Design review of the part built by this model. Coordinates are the model's own, in mm. A direction names the side the tool comes from. Coordinates: 2 decimals unless noted, no trailing zeros. Write each loop counter-clockwise with the first axis right and the second up, starting at its lowest first coordinate (ties: lowest second). Pieces come first, ordered by that corner, then holes. Notation, with made-up numbers: (-14.75, -30) - (-9.75, -30) arc R26 cw to (-9.75, 6) - close; hole circle Ø5 at (58, 17). An arc over 180 degrees is marked (long way). One line per item, written item: value.
from build123d import *

# Parameters (mm, degrees)
F0_R     = 10.16
F1_DEPTH = 15.7734
F3_DEPTH = 25.4
F4_R     = 5.08


with BuildPart() as f1:
    # F0 (on Top) → F1 (new body)
    with BuildSketch(Plane.XY):
        with BuildLine():
            ThreePointArc((5.0426470588, -28.1265414802), (21.9160245563, -18.3362616868), (28.575, 0))
            ThreePointArc((28.575, 0), (21.9160245563, 18.3362616868), (5.0426470588, 28.1265414802))
            ThreePointArc((5.0426470588, 28.1265414802), (-28.575, 0), (5.0426470588, -28.1265414802))
        make_face()
        with BuildLine():
            ThreePointArc((13.4477648793, -4.826), (-14.2875, 0), (13.4477648793, 4.826))
            Line((13.4477648793, 4.826), (18.5293, 4.826))
            Line((18.5293, 4.826), (18.5293, -4.826))
            Line((18.5293, -4.826), (13.4477648793, -4.826))
        make_face(mode=Mode.SUBTRACT)
        with BuildLine():
            ThreePointArc((5.0426470588, 28.1265414802), (21.9160245563, 18.3362616868), (28.575, 0))
            ThreePointArc((28.575, 0), (21.9160245563, -18.3362616868), (5.0426470588, -28.1265414802))
            Line((5.0426470588, -28.1265414802), (57.3367647059, -18.7510276535))
            ThreePointArc((57.3367647059, -18.7510276535), (73.025, 0), (57.3367647059, 18.7510276535))
            Line((57.3367647059, 18.7510276535), (5.0426470588, 28.1265414802))
        make_face()
        with Locations((53.975, 0)):
            Circle(F0_R, mode=Mode.SUBTRACT)
    extrude(amount=F1_DEPTH)

    # F2 (on face) → F3 (join)
    with BuildSketch(Plane.XY.offset(15.7734)):
        with BuildLine():
            ThreePointArc((5.0426470588, -28.1265414802), (21.9160245563, -18.3362616868), (28.575, 0))
            ThreePointArc((28.575, 0), (21.9160245563, 18.3362616868), (5.0426470588, 28.1265414802))
            ThreePointArc((5.0426470588, 28.1265414802), (-28.575, 0), (5.0426470588, -28.1265414802))
        make_face()
        with BuildLine():
            Line((18.5293, -4.826), (13.4477648793, -4.826))
            ThreePointArc((13.4477648793, -4.826), (-14.2875, 0), (13.4477648793, 4.826))
            Line((13.4477648793, 4.826), (18.5293, 4.826))
            Line((18.5293, 4.826), (18.5293, -4.826))
        make_face(mode=Mode.SUBTRACT)
    extrude(amount=F3_DEPTH)

    # F4
    f4_edges = [f1.edges().sort_by_distance(p)[0] for p in [
        (-5.042647, 28.126541, 41.1734),
    ]]
    fillet(f4_edges, radius=F4_R)


solid = f1.part
1. Wall thickness on line 1 along X through (y, z) = (0, 30) (1 decimal); line 2 along Y through (x, z) = (0, 33.5) (1 decimal); line 3 along Z through (x, y) = (38, 9.5): over which ranges is each line inside the solid? List them lowest first.
Answer block:
line 1: x = -28.6 to -14.3, 18.5 to 28.6
line 2: y = -28.6 to -14.3, 14.3 to 28.6
line 3: z = 0 to 15.77
2. Consider section A-A, the plane z = 3. Give the number of separate pieces and of enclosed holes in the cut face, then the cut area to 3 significant figures.
Answer block:
separate pieces: 1
enclosed holes: 2
area: 3,450 mm^2
3. Consider section B-B, the plane x = 56. Write out the cut boundary in (y, z).
Answer block:
outline: (-18.99, 0) - (-9.96, 0) - (-9.96, 15.77) - (-18.99, 15.77) - close; (9.96, 0) - (18.99, 0) - (18.99, 15.77) - (9.96, 15.77) - close
4. Insertion check: pin 1 Ø5 at (x, z) = (46.5, 8) entering from +Y; pin 2 Ø2.5 at (x, z) = (16, 14.5) entering from -Y; pin 3 Ø6 at (x, y) = (6, -8.5) entering from +Z; pin 4 Ø2.5 at (x, z) = (16.5, 16.5) entering from +Y. Each pin has a flat end and moves straight along its axis. Give the tip position at first contact, or say it passes through.
Answer block:
pin 1: stops at y = 21.14
pin 2: stops at y = -26.39
pin 3: passes through
pin 4: stops at y = 26.25
5. Mouldability with a two-part tool opening along Y and no side actions: class faces 1 (the face through (31.556, 23.373, 7.776)), 2 (the face through (73.02, -0.37, 7.78)), 3 (the face through (-14.277, -0.559, 20.298)) as released by +Y, released by -Y, zero draft, split by the parting line, or undercut.
Answer block:
face 1: released by +Y
face 2: split by the parting line
face 3: undercut
6. For faces 4 (the face through (18.529, 0, 20)), 5 (the face through (30.824, -23.504, 7.776)), list the 3-axis set-ups (+Z, -Z, +X, -X, +Y, -Y) from which the entire face can be reached by the end or side of a thin tool; tool diameter is ignored.
Answer block:
face 4: +Z, -Z
face 5: +Z, -Z, +X, -Y
